from build123d import *

# Parameters (mm, degrees)
SKETCH3_W           = 120
SKETCH3_H           = 150
BOSS_EXTRUDE2_DEPTH = 5
BOSS_EXTRUDE3_DEPTH = 45
SKETCH5_W           = 110
SKETCH5_H           = 150
BOSS_EXTRUDE4_DEPTH = 5
SKETCH6_R           = 6.5
CUT_EXTRUDE1_DEPTH  = 5
SKETCH7_W           = 40
SKETCH7_H           = 140
BOSS_EXTRUDE5_DEPTH = 8
SKETCH8_W           = 40
SKETCH8_H           = 5
BOSS_EXTRUDE6_DEPTH = 25.5
SKETCH9_R           = 1.5
CUT_EXTRUDE2_DEPTH  = 10
SKETCH10_W          = 47.5
SKETCH10_H          = 8
CUT_EXTRUDE3_DEPTH  = 40
SKETCH11_W          = 45
SKETCH11_H          = 33.5
CUT_EXTRUDE4_DEPTH  = 40
SKETCH12_W          = 56
SKETCH12_H          = 15
BOSS_EXTRUDE7_DEPTH = 40
SKETCH13_W          = 7
SKETCH13_H          = 20.5
BOSS_EXTRUDE8_DEPTH = 11
SKETCH14_W          = 56
SKETCH14_H          = 5
BOSS_EXTRUDE9_DEPTH = 11


with BuildPart() as part:
    # Sketch3 → Boss-Extrude2 (new body)
    with BuildSketch(Plane(origin=(0, 0, 0), x_dir=(1, 0, 0), z_dir=(0, 1, 0))):
        with Locations((60, 75)):
            Rectangle(SKETCH3_W, SKETCH3_H)
    extrude(amount=BOSS_EXTRUDE2_DEPTH)

    # Sketch4 → Boss-Extrude3 (add)
    with BuildSketch(Plane(origin=(0, 5, 0), x_dir=(1, 0, 0), z_dir=(0, 1, 0))):
        Polygon((10, 0), (10, 5), (115, 5), (115, 145), (10, 145), (10, 150), (120, 150), (120, 0), align=None)
    extrude(amount=BOSS_EXTRUDE3_DEPTH)

    # Sketch5 → Boss-Extrude4 (add)
    with BuildSketch(Plane(origin=(0, 50, 0), x_dir=(1, 0, 0), z_dir=(0, 1, 0))):
        with Locations((65, 75)):
            Rectangle(SKETCH5_W, SKETCH5_H)
    extrude(amount=BOSS_EXTRUDE4_DEPTH)

    # Sketch6 → Cut-Extrude1 (cut)
    with BuildSketch(Plane(origin=(120, 0, 0), x_dir=(0, 0, -1), z_dir=(1, 0, 0))):
        with Locations((75, 30)):
            Circle(SKETCH6_R)
    extrude(amount=-CUT_EXTRUDE1_DEPTH, mode=Mode.SUBTRACT)

    # Sketch7 → Boss-Extrude5 (add)
    with BuildSketch(Plane(origin=(0, 5, 0), x_dir=(1, 0, 0), z_dir=(0, 1, 0))):
        with Locations((95, 75)):
            Rectangle(SKETCH7_W, SKETCH7_H)
    extrude(amount=BOSS_EXTRUDE5_DEPTH)

    # Sketch8 → Boss-Extrude6 (add)
    with BuildSketch(Plane(origin=(0, 13, 0), x_dir=(1, 0, 0), z_dir=(0, 1, 0))):
        with Locations((95, 55)):
            Rectangle(SKETCH8_W, SKETCH8_H)
        with Locations((95, 95)):
            Rectangle(SKETCH8_W, SKETCH8_H)
    extrude(amount=BOSS_EXTRUDE6_DEPTH)

    # Sketch9 → Cut-Extrude2 (cut)
    with BuildSketch(Plane.ZY.offset(-10)):
        with Locations((-147.5, 10)):
            Circle(SKETCH9_R)
        with Locations((-147.5, 52.5)):
            Circle(SKETCH9_R)
        with Locations((-2.5, 10)):
            Circle(SKETCH9_R)
        with Locations((-2.5, 52.5)):
            Circle(SKETCH9_R)
    extrude(amount=-CUT_EXTRUDE2_DEPTH, mode=Mode.SUBTRACT)

    # Sketch10 → Cut-Extrude3 (cut)
    with BuildSketch(Plane.ZY.offset(-75)):
        with Locations((-121.25, 9)):
            Rectangle(SKETCH10_W, SKETCH10_H)
        with Locations((-28.75, 9)):
            Rectangle(SKETCH10_W, SKETCH10_H)
    extrude(amount=-CUT_EXTRUDE3_DEPTH, mode=Mode.SUBTRACT)

    # Sketch11 → Cut-Extrude4 (cut)
    with BuildSketch(Plane.ZY.offset(-75)):
        with Locations((-75, 21.75)):
            Rectangle(SKETCH11_W, SKETCH11_H)
    extrude(amount=-CUT_EXTRUDE4_DEPTH, mode=Mode.SUBTRACT)

    # Sketch12 → Boss-Extrude7 (add)
    with BuildSketch(Plane.ZY.offset(-115)):
        with Locations((-64.5, 12.5)):
            Rectangle(SKETCH12_W, SKETCH12_H)
    extrude(amount=BOSS_EXTRUDE7_DEPTH)

    # Sketch13 → Boss-Extrude8 (add)
    with BuildSketch(Plane.ZY.offset(-115)):
        with Locations((-89, 30.25)):
            Rectangle(SKETCH13_W, SKETCH13_H)
        with Locations((-40, 30.25)):
            Rectangle(SKETCH13_W, SKETCH13_H)
    extrude(amount=BOSS_EXTRUDE8_DEPTH)

    # Sketch14 → Boss-Extrude9 (add)
    with BuildSketch(Plane.ZY.offset(-115)):
        with Locations((-64.5, 43)):
            Rectangle(SKETCH14_W, SKETCH14_H)
    extrude(amount=BOSS_EXTRUDE9_DEPTH)


solid = part.part
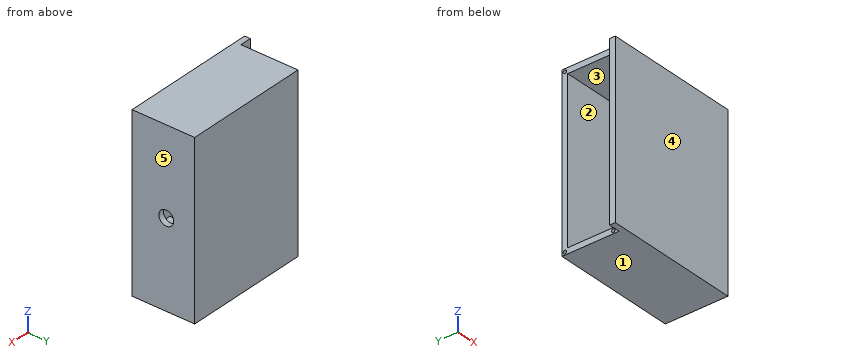
The listing builds one solid part. Answer for the finished solid, in the listing's coordinates (mm). Face numbers are marked on the shaded views. A direction names the side the tool comes from. Coordinates: 2 decimals unless noted, no trailing zeros. Write each loop counter-clockwise with the first axis right and the second up, starting at its lowest first coordinate (ties: lowest second). Pieces come first, ordered by that corner, then holes. Notation, with made-up numbers: (-7.5, 36) -> (13.5, 36) arc R23 cw to (13.5, 65) -> close; hole circle Ø4 at (57.5, 52.5). An arc over 180 degrees is marked (long way). One line per question, with ' | ' between items.
1. Section B-B (z = -75) is taken. Determine the outline of the cut face in (x, y).
Verdict:
outline: (0, 0) -> (120, 0) -> (120, 23.5) -> (115, 23.5) -> (115, 20) -> (75, 20) -> (75, 5) -> (0, 5) -> close; (10, 50) -> (115, 50) -> (115, 45.5) -> (104, 45.5) -> (104, 40.5) -> (115, 40.5) -> (115, 36.5) -> (120, 36.5) -> (120, 55) -> (10, 55) -> close
2. Section A-A (x = 58) is taken. Determine the outline of the cut face in (y, z).
Verdict:
outline: (0, -150) -> (55, -150) -> (55, 0) -> (0, 0) -> close; hole (5, -145) -> (50, -145) -> (50, -5) -> (5, -5) -> close
3. Straight lines are drawn through the part: line 1 (Z direction, x = 79.5, y = 17.5); line 2 (Z direction, x = 105.5, y = 22); line 3 (Y direction, x = 13, z = -2.5). For each, find the intervals that lie inside material, in ascending order.
Verdict:
line 1: z = -150 to -145, -92.5 to -36.5, -5 to 0 | line 2: z = -150 to -145, -92.5 to -85.5, -43.5 to -36.5, -5 to 0 | line 3: y = 0 to 8.5, 11.5 to 51, 54 to 55
4. Section D-D (z = -111) is taken. Determine the outline of the cut face in (x, y), and give its area (4 significant figures).
Verdict:
outline: (0, 0) -> (120, 0) -> (120, 55) -> (10, 55) -> (10, 50) -> (115, 50) -> (115, 5) -> (0, 5) -> close | area: 1,375 mm^2
5. Section C-C (y = 30) is taken. Determine the outline of the cut face in (x, z), and give its area (3 significant figures).
Verdict:
outline: (10, -150) -> (120, -150) -> (120, -81.5) -> (115, -81.5) -> (115, -85.5) -> (104, -85.5) -> (104, -92.5) -> (115, -92.5) -> (115, -145) -> (10, -145) -> close; (10, -5) -> (115, -5) -> (115, -36.5) -> (104, -36.5) -> (104, -43.5) -> (115, -43.5) -> (115, -68.5) -> (120, -68.5) -> (120, 0) -> (10, 0) -> close | area: 1,890 mm^2
6. Given pin 1 Ø1.5 at (y, z) = (10.5, -148) entering from -X; pin 2 Ø6 at (y, z) = (13.5, -66) entering from -X, each flat-ended and moving along its own axis, determine where each tip first touches the part or whether it passes through.
Verdict:
pin 1: stops at x = 20 | pin 2: stops at x = 75
7. For a pull along Y with two mould halves and no side action, classify the marked faces 3, 4 and 5 as released by +Y, released by -Y, zero draft, split by the parting line, or undercut.
Verdict:
face 3: undercut | face 4: released by -Y | face 5: zero draft
8. Which of the six approach directions +Z, -Z, +X, -X, +Y, -Y give full straight-line access (tool end or side, diameter ignored) to the marked faces 1 and 2?
Verdict:
face 1: -Z, +X, -X, +Y, -Y | face 2: -X
